Input: part model. Units: mm. Frame: model coordinates. A direction names the side the tool comes from. Give positions to 0.01 mm unless a question says otherwise; leave off trailing zeros. Loops run counter-clockwise (first coordinate to the right, second up) from the corner with the lowest first, then second, coordinate; pieces in that order, holes last. Notation, with made-up numbers: (42, 14) -> (87, 14) arc R30 cw to (87, 47) -> close; hole circle Ø9 at (45, -34). An arc over 180 degrees is marked (long way). Use CSV: the item, a comma, the result in double quotes.
```python
from build123d import *

# Parameters (mm, degrees)
F0_R     = 43.18
F1_DEPTH = 25.4
F2_R     = 17.018
F3_DEPTH = 27.686
F4_R     = 35.7378
F5_DEPTH = 23.876
F6_R     = 17.783097


with BuildPart() as f1:
    # F0 (on Top) → F1 (new body)
    with BuildSketch(Plane.XY):
        Circle(F0_R)
    extrude(amount=F1_DEPTH)

    # F2 (on face) → F3 (cut)
    with BuildSketch(Plane.XY):
        Circle(F2_R)
    extrude(amount=F3_DEPTH, mode=Mode.SUBTRACT)

    # F4 (on face) → F5 (cut)
    with BuildSketch(Plane.XY.offset(25.4)):
        Circle(F4_R)
    extrude(amount=-F5_DEPTH, mode=Mode.SUBTRACT)

    # F6
    f6_edges = [f1.edges().sort_by_distance(p)[0] for p in [
        (-35.7378, 0, 1.524),
    ]]
    fillet(f6_edges, radius=F6_R)


solid = f1.part
```
1) Reachability of faces 1 (the flat face through (-16.2, 32.2, 25.4)), 2 (the cylindrical face through (-7.7, -34.9, 22.4)) from +Z, -Z, +X, -X, +Y, -Y: full face, straight path, thin tool, end or side. Return the list, or none.
From the geometry:
face 1,"+Z, +X, -X, +Y, -Y"
face 2,"+Z"
2) Mould query, pull axis Y, two halves, no side actions, for faces 3 (the flat face through (16, -7, 1.524)), 4 (the flat face through (19, 1, 0)), 5 (the cylindrical face through (-31.83, 29.18, 12.52)). Classes: pulls with the +Y half, pulls with the -Y half, needs draft (parallel to the pull), parting line crosses it, or undercut.
From the geometry:
face 3,"undercut"
face 4,"needs draft"
face 5,"parting line crosses it"
3) Section query C-C (z = 21.5). Return loops of the section in (x, y).
From the geometry:
outline,"circle Ø86.36 at (0, 0); hole circle Ø71.48 at (0, 0)"
4) Contact query for flat-ended pins moving along their axis: pin 1 (5 mm diameter, centred on x = -2.5, y = 26.5, fed in from +Z); pin 2 (1.5 mm diameter, centred on x = -32.5, y = -25.5, fed in from -Z); pin 3 (3 mm diameter, centred on x = -20, y = -17.5, fed in from +Z); pin 4 (6 mm diameter, centred on x = -15.5, z = 22, fed in from -Y). Output: stop coordinate, or through.
From the geometry:
pin 1,"stops at z = 5.46"
pin 2,"stops at z = 0"
pin 3,"stops at z = 4.68"
pin 4,"stops at y = -41.33"
5) Ray query, line 1 (Y direction, x = 0, z = 1.05); line 2 (Y direction, x = 0, z = 22.75); line 3 (X direction, y = -18.5, z = 14.5). Return the intervals inside material, ascending.
From the geometry:
line 1,"y = -43.18 to -17.02, 17.02 to 43.18"
line 2,"y = -43.18 to -35.74, 35.74 to 43.18"
line 3,"x = -39.02 to -29.8, 29.8 to 39.02"
6) Section query D-D (z = 16.25). Return loops of the section in (x, y).
From the geometry:
outline,"circle Ø86.36 at (0, 0); hole circle Ø70.95 at (0, 0)"
7) Section query A-A (x = 0). Return loops of the section in (y, z).
From the geometry:
outline,"(-43.18, 0) -> (-17.02, 0) -> (-17.02, 1.52) -> (-17.95, 1.52) arc R17.78 cw to (-35.74, 19.31) -> (-35.74, 25.4) -> (-43.18, 25.4) -> close; (17.02, 0) -> (43.18, 0) -> (43.18, 25.4) -> (35.74, 25.4) -> (35.74, 19.31) arc R17.78 cw to (17.95, 1.52) -> (17.02, 1.52) -> close"
